Geometry check sheet. Reference: the model listing, model coordinates, mm. Coordinates: 2 decimals unless noted, no trailing zeros. Write each loop counter-clockwise with the first axis right and the second up, starting at its lowest first coordinate (ties: lowest second). Pieces come first, ordered by that corner, then holes. Notation, with made-up numbers: (87.25, 64.5) -> (109.25, 64.5) arc R10 cw to (109.25, 80.5) -> close; hole circle Ø5 at (65, 74). An arc over 180 degrees is marked (long way). Use a Markdown table: item, result.
```python
from build123d import *

# Parameters (mm, degrees)
SKETCH1_W           = 45.2
SKETCH1_H           = 20.6
BOSS_EXTRUDE1_DEPTH = 1.1
SKETCH18_R          = 1
CUT_EXTRUDE4_DEPTH  = 2.1
SKETCH30_R          = 0.15
CUT_EXTRUDE6_DEPTH  = 1.1


with BuildPart() as part:
    # Sketch1 → Boss-Extrude1 (new body)
    with BuildSketch(Plane(origin=(0, 0, 0), x_dir=(1, 0, 0), z_dir=(0, 1, 0))):
        Rectangle(SKETCH1_W, SKETCH1_H)
    extrude(amount=BOSS_EXTRUDE1_DEPTH)

    # Sketch18 → Cut-Extrude4 (cut, through all)
    with BuildSketch(Plane(origin=(0, 1.1, 0), x_dir=(1, 0, 0), z_dir=(0, 1, 0))):
        with Locations((-21.2, -8.9)):
            Circle(SKETCH18_R)
        with Locations((21.2, 8.9)):
            Circle(SKETCH18_R)
    cut_extrude4 = extrude(amount=-CUT_EXTRUDE4_DEPTH, mode=Mode.SUBTRACT)

    # Sketch30 → Cut-Extrude6 (cut)
    with BuildSketch(Plane.XZ):
        with Locations((-9.333130036, 4.387708864)):
            Circle(SKETCH30_R)
        with Locations((-8.744545033, 3.449056667)):
            Circle(SKETCH30_R)
        with Locations((4.759894179, 5.015066472)):
            Circle(SKETCH30_R)
        with Locations((16.922953898, 5.247379324)):
            Circle(SKETCH30_R)
        with Locations((7.830601522, -1.527883327)):
            Circle(SKETCH30_R)
        with Locations((7.85211857, -0.548857679)):
            Circle(SKETCH30_R)
        with Locations((5.549794517, -2.808147637)):
            Circle(SKETCH30_R)
        with Locations((5.883308749, 1.656639662)):
            Circle(SKETCH30_R)
        with Locations((15.827488091, -3.115541656)):
            Circle(SKETCH30_R)
        with Locations((21.375936622, -3.969149123)):
            Circle(SKETCH30_R)
        with Locations((17.961506757, -7.584427803)):
            Circle(SKETCH30_R)
        with Locations((15.35602841, -9.449889168)):
            Circle(SKETCH30_R)
        with Locations((3.599221967, -6.119367867)):
            Circle(SKETCH30_R)
        with Locations((7.740262146, -8.603991974)):
            Circle(SKETCH30_R)
        with Locations((-0.570878142, -8.77835156)):
            Circle(SKETCH30_R)
        with Locations((-2.901654637, -4.656320507)):
            Circle(SKETCH30_R)
        with Locations((-4.176494296, -4.656320507)):
            Circle(SKETCH30_R)
        with Locations((-5.415606667, -1.349023089)):
            Circle(SKETCH30_R)
        with Locations((-7.901413801, -0.278896563)):
            Circle(SKETCH30_R)
        with Locations((-5.254994429, 5.1458063)):
            Circle(SKETCH30_R)
        with Locations((-3.895298753, 7.064281021)):
            Circle(SKETCH30_R)
        with Locations((13.574528056, 2.494833551)):
            Circle(SKETCH30_R)
        with Locations((10.060923878, 0.512200964)):
            Circle(SKETCH30_R)
        with Locations((-12.870283271, -7.223609825)):
            Circle(SKETCH30_R)
        with Locations((-20.003938885, -5.491150605)):
            Circle(SKETCH30_R)
        with Locations((-22.357061828, 3.218671023)):
            Circle(SKETCH30_R)
        with Locations((-22.357061828, 1.95517224)):
            Circle(SKETCH30_R)
        with Locations((-22.357061828, -1.948730844)):
            Circle(SKETCH30_R)
    extrude(amount=-CUT_EXTRUDE6_DEPTH, mode=Mode.SUBTRACT)

    # Mirror1: Cut-Extrude4 across plane
    add(cut_extrude4.mirror(Plane(origin=(0, 0, 0), x_dir=(0, 0, 1), z_dir=(1, 0, 0))), mode=Mode.SUBTRACT)


solid = part.part
```
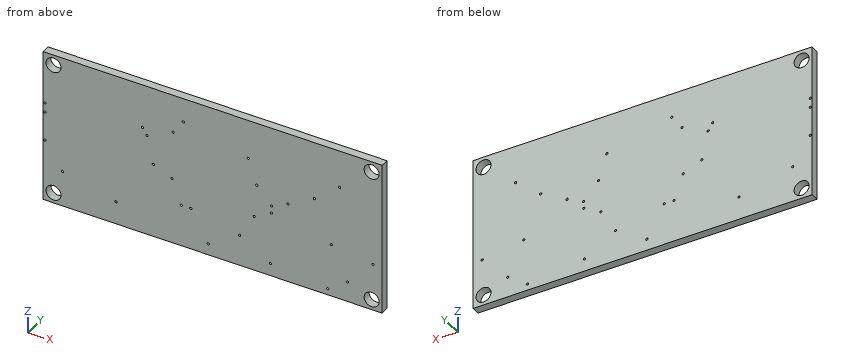
Item 1: Section check B-B on x = -21.2. Record the boundary of the cut face in (y, z), then the cut area to 3 significant figures.
Answer block:
| item | result |
|---|---|
| outline | (0, -10.3) -> (1.1, -10.3) -> (1.1, -9.9) -> (0, -9.9) -> close; (0, -7.9) -> (1.1, -7.9) -> (1.1, 7.9) -> (0, 7.9) -> close; (0, 9.9) -> (1.1, 9.9) -> (1.1, 10.3) -> (0, 10.3) -> close |
| area | 18.3 mm^2 |
Item 2: Section check C-C on y = 0.3. Count the separate pieces of the cut face and the enclosed holes in it, then the cut area to 3 significant figures.
Answer block:
| item | result |
|---|---|
| separate pieces | 1 |
| enclosed holes | 32 |
| area | 917 mm^2 |
Item 3: Section check A-A on z = 8.9. Record the boundary of the cut face in (x, y).
Answer block:
| item | result |
|---|---|
| outline | (-22.6, 0) -> (-22.2, 0) -> (-22.2, 1.1) -> (-22.6, 1.1) -> close; (-20.2, 0) -> (20.2, 0) -> (20.2, 1.1) -> (-20.2, 1.1) -> close; (22.2, 0) -> (22.6, 0) -> (22.6, 1.1) -> (22.2, 1.1) -> close |
Item 4: Depth check by flat-ended pin: P1, Ø1.2, axis at x = 21.2, z = 8.9, coming from the -Y side. Enter the tip coordinate at first touch or a pass-through.
Answer block:
| item | result |
|---|---|
| P1 | passes through |
Item 5: Thickness scan on L1, parallel to X at y = 1, z = -0.5; L2, parallel to Z at x = -20, y = 0.65; L3, parallel to X at y = 0.2, z = -5.5. Record the ranges inside material, lowest first. Write a range as [from, to].
Answer block:
| item | result |
|---|---|
| L1 | x = [-22.6, 7.71], [7.99, 22.6] |
| L2 | z = [-10.3, -5.64], [-5.34, 10.3] |
| L3 | x = [-22.6, -20.15], [-19.85, 22.6] |
